Here's the drawing with two shaded views (mm, measured from the low corner). I have some questions. Give positions to 0.01 mm unless a question says otherwise; leave off trailing zeros. Write each loop counter-clockwise with the first axis right and the second up, starting at its lowest first coordinate (ties: lowest second). Pieces come first, ordered by that corner, then holes. Notation, with made-up numbers: M 78.25,82 L 90.25,82 A22 cw 90.25,91 Z; hole C 5.5,0.25 d6. An arc over 180 degrees is marked long. Answer as CSV lines item,"result". Start each with the question number.
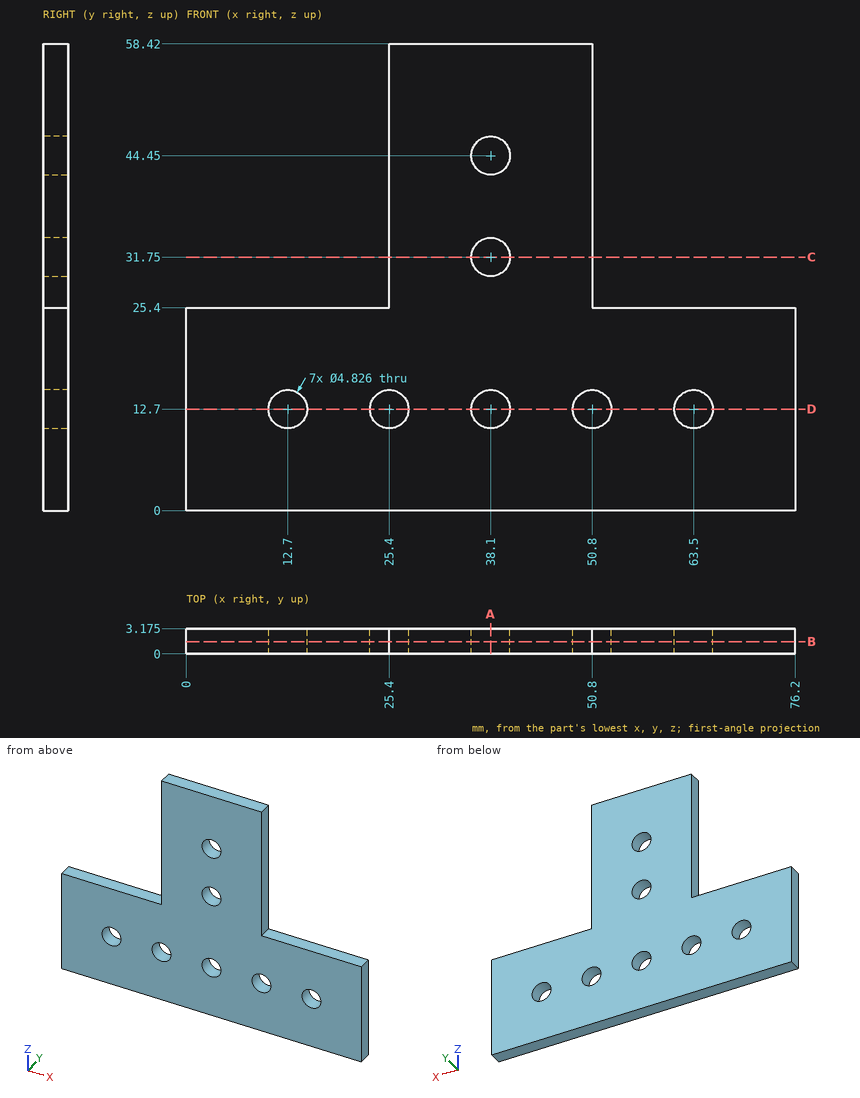
1. Imagine slicing it at D-D, the plane z = 12.7. Please give me the cut outline in (x, y) (3 decimals).
2. Will these pins go through, and if not, where does the flat tip stop? P1, Ø5.5, axis at x = 38.1, z = 12.7, coming from the -Y side; P2, Ø1.6, axis at x = 62, y = 1.5, coming from the +Z side; P3, Ø1, axis at y = 2, z = 35.5, coming from the +X side; P4, Ø1.6, axis at y = 1.5, z = 49, coming from the -X side.
3. Please list where these lines run through material, in increasing order: line 1 (X direction, y = 2, z = 12.7); line 2 (Z direction, x = 38.1, y = 1.4); line 3 (Z direction, x = 19, y = 2.6).
4. Imagine slicing it at B-B, the plane y = 1.55. Please give me the cut outline in (x, z).
5. Imagine slicing it at A-A, the plane x = 38.1. Please give me the cut outline in (y, z) (3 decimals).
6. Imagine slicing it at C-C, the plane z = 31.75. Please give me the cut outline in (x, y) (3 decimals).
Solutions:
1,outline,"M 0,0 L 10.287,0 L 10.287,3.175 L 0,3.175 Z; M 15.113,0 L 22.987,0 L 22.987,3.175 L 15.113,3.175 Z; M 27.813,0 L 35.687,0 L 35.687,3.175 L 27.813,3.175 Z; M 40.513,0 L 48.387,0 L 48.387,3.175 L 40.513,3.175 Z; M 53.213,0 L 61.087,0 L 61.087,3.175 L 53.213,3.175 Z; M 65.913,0 L 76.2,0 L 76.2,3.175 L 65.913,3.175 Z"
2,P1,"y = 0"
2,P2,"z = 25.4"
2,P3,"x = 50.8"
2,P4,"x = 25.4"
3,line 1,"0 to 10.29, 15.11 to 22.99, 27.81 to 35.69, 40.51 to 48.39, 53.21 to 61.09, 65.91 to 76.2"
3,line 2,"0 to 10.29, 15.11 to 29.34, 34.16 to 42.04, 46.86 to 58.42"
3,line 3,"0 to 25.4"
4,outline,"M 0,0 L 76.2,0 L 76.2,25.4 L 50.8,25.4 L 50.8,58.42 L 25.4,58.42 L 25.4,25.4 L 0,25.4 Z; hole C 12.7,12.7 d4.83; hole C 25.4,12.7 d4.83; hole C 38.1,12.7 d4.83; hole C 38.1,31.75 d4.83; hole C 38.1,44.45 d4.83; hole C 50.8,12.7 d4.83; hole C 63.5,12.7 d4.83"
5,outline,"M 0,0 L 3.175,0 L 3.175,10.287 L 0,10.287 Z; M 0,15.113 L 3.175,15.113 L 3.175,29.337 L 0,29.337 Z; M 0,34.163 L 3.175,34.163 L 3.175,42.037 L 0,42.037 Z; M 0,46.863 L 3.175,46.863 L 3.175,58.42 L 0,58.42 Z"
6,outline,"M 25.4,0 L 35.687,0 L 35.687,3.175 L 25.4,3.175 Z; M 40.513,0 L 50.8,0 L 50.8,3.175 L 40.513,3.175 Z"
